For this review, use the dimensioned drawing (mm, ordinates from the lowest corner) and the shaded views. Coordinates: 2 decimals unless noted, no trailing zeros. Order: outer loops, then holes, each group sorted by start corner. A loop starts at its lowest first (then second) coordinate and runs counter-clockwise, first axis right, second up. Notation, with made-up numbers: M 10.25,-34 L 38.25,-34 A19 cw 38.25,-4 Z; hole C -25,3.25 d1. An arc over 180 degrees is marked long. Answer in a Markdown table with one row per item.
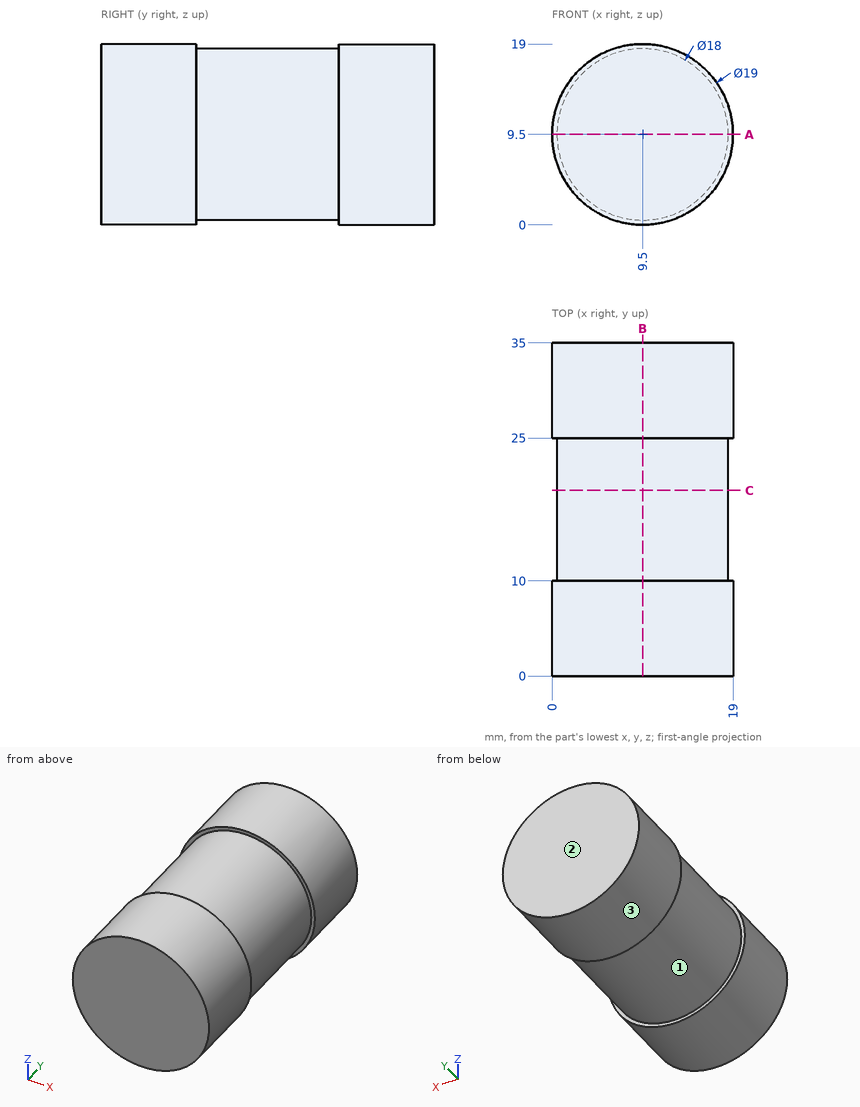
(1) Add section A-A, the plane z = 9.5. Give the boundary of the cut face in (x, y), and give its area (3 significant figures).
Return value:
| item | result |
|---|---|
| outline | M 0,0 L 19,0 L 19,10 L 18.5,10 L 18.5,25 L 19,25 L 19,35 L 0,35 L 0,25 L 0.5,25 L 0.5,10 L 0,10 Z |
| area | 650 mm2 |
(2) Draft analysis for pull direction Y (two halves, no side actions). For the marked faces 1, 2 and 3, state which applies: pulls with the +Y half, pulls with the -Y half, needs draft (parallel to the pull), parting line crosses it, or undercut.
Return value:
| item | result |
|---|---|
| face 1 | undercut |
| face 2 | pulls with the +Y half |
| face 3 | needs draft |
(3) Insertion check: pin 1 Ø6 at (x, y) = (5, 18) entering from +Z; pin 2 Ø1.5 at (y, z) = (27, 4.5) entering from +X; pin 3 Ø1.5 at (y, z) = (29, 4.5) entering from -X. Each pin has a flat end and moves straight along its axis. Give the tip position at first contact, or say it passes through.
Return value:
| item | result |
|---|---|
| pin 1 | stops at z = 18.37 |
| pin 2 | stops at x = 18 |
| pin 3 | stops at x = 1 |
(4) For line 1 along X through (y, z) = (3, 9.75); line 2 along Y through (x, z) = (2, 14.75); line 3 along X through (y, z) = (21, 9.25), list the stretches that pass through material, from the lowest coordinate up. Write a range as from..to.
Return value:
| item | result |
|---|---|
| line 1 | x = 0..19 |
| line 2 | y = 0..10, 25..35 |
| line 3 | x = 0.5..18.5 |
(5) Add section C-C, the plane y = 19.5. Give the boundary of the cut face in (x, z), and give its area (3 significant figures).
Return value:
| item | result |
|---|---|
| outline | C 9.5,9.5 d18 |
| area | 254 mm2 |
(6) Add section B-B, the plane x = 9.5. Give the boundary of the cut face in (y, z).
Return value:
| item | result |
|---|---|
| outline | M 0,0 L 10,0 L 10,0.5 L 25,0.5 L 25,0 L 35,0 L 35,19 L 25,19 L 25,18.5 L 10,18.5 L 10,19 L 0,19 Z |
